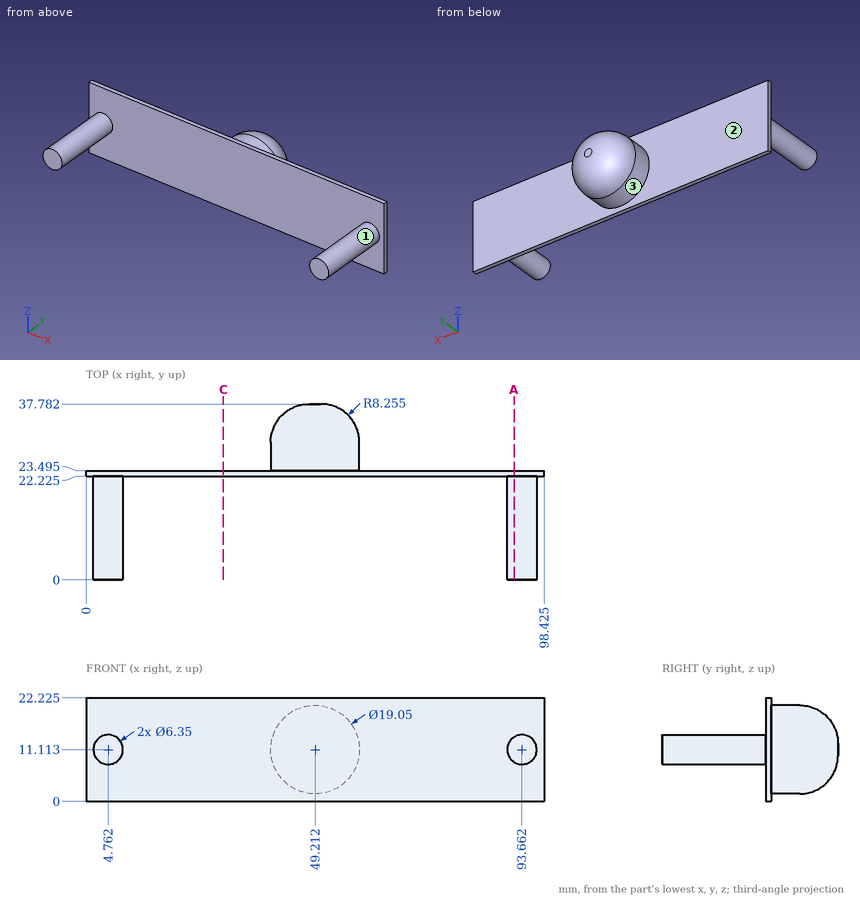
Input: dimensioned drawing with shaded views. Units: mm. Origin: part minimum x, y, z. Round coordinates to 2 decimals unless told otherwise and drop trailing zeros. Order: outer loops, then holes, each group sorted by start corner. A loop starts at its lowest first (then second) coordinate and runs counter-clockwise, first axis right, second up.
1. Material intervals for line 1 (X direction, y = 20, z = 11.25) (1 decimal); line 2 (Y direction, x = 40, z = 19) (1 decimal); line 3 (X direction, y = 15, z = 12) (1 decimal), sorted ascending.
The answers:
line 1: x = 1.6 to 7.9, 90.5 to 96.8
line 2: y = 22.2 to 23.5
line 3: x = 1.7 to 7.8, 90.6 to 96.7
2. Cut plane C-C, the plane x = 29.5. Output: boundary loops of the cut face in (y, z) (1 decimal).
The answers:
outline: (22.2, 0) - (23.5, 0) - (23.5, 22.2) - (22.2, 22.2) - close
3. Pin query (flat end, axial travel): P1, Ø10, axis at y = 33.5, z = 16.5, coming from the -X side; P2, Ø10, axis at y = 34, z = 12.5, coming from the +X side; P3, Ø1.5, axis at x = 13.5, z = 18, coming from the +Y side (1 decimal). Return the tip coordinate at first contact, or that it passes through.
The answers:
P1: stops at x = 39.85
P2: stops at x = 58.74
P3: stops at y = 23.5
4. Cut plane A-A, the plane x = 92. Output: boundary loops of the cut face in (y, z) (1 decimal).
The answers:
outline: (0, 8.4) - (22.2, 8.4) - (22.2, 0) - (23.5, 0) - (23.5, 22.2) - (22.2, 22.2) - (22.2, 13.8) - (0, 13.8) - close
5. Mould query, pull axis X, two halves, no side actions, for the marked faces 1, 2 and 3. Classes: released by +X, released by -X, zero draft, split by the parting line, or undercut.
The answers:
face 1: undercut
face 2: zero draft
face 3: split by the parting line
